from build123d import *

# Parameters (mm, degrees)
F2_R     = 11.5
F2_R_2   = 10
F3_DEPTH = 16
F4_DEPTH = 1.5
F5_R     = 0.3
F6_SIZE2 = 0.3
F6_SIZE  = 2


with BuildPart() as f3:
    # F2 (on Top) → F3 (new body)
    with BuildSketch(Plane.XY):
        Circle(F2_R)
        Circle(F2_R_2, mode=Mode.SUBTRACT)
    extrude(amount=F3_DEPTH)

    # F2 (on Top) → F4 (join)
    with BuildSketch(Plane.XY):
        Circle(F2_R_2)
    extrude(amount=F4_DEPTH)

    # F5
    f5_edges = [f3.edges().sort_by_distance(p)[0] for p in [
        (-11.5, 0, 0),
    ]]
    fillet(f5_edges, radius=F5_R)

    # F6
    f6_edges = [f3.edges().sort_by_distance(p)[0] for p in [
        (-10, 0, 16),
    ]]
    f6_side = f3.faces().sort_by_distance((-10, 0, 8.75))[0]
    chamfer(f6_edges, length=F6_SIZE, length2=F6_SIZE2, reference=f6_side)


solid = f3.part
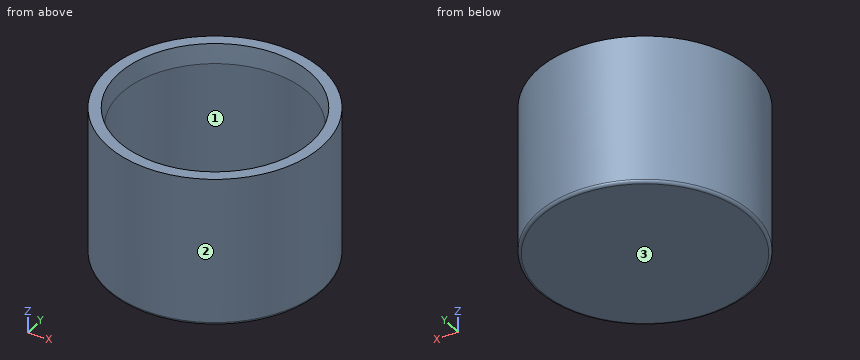
Could you check a few things on this model? Use its own coordinates, in mm. Face numbers are marked on the shaded views. Give positions to 0.01 mm unless a question says otherwise; leave off trailing zeros. Write each loop counter-clockwise with the first axis right and the second up, starting at its lowest first coordinate (ties: lowest second). Pieces come first, ordered by that corner, then holes. Notation, with made-up numbers: (-16.75, -5.5) -> (29.25, -5.5) arc R9 cw to (29.25, 6.5) -> close; hole circle Ø9 at (79.5, 62). An arc over 180 degrees is marked (long way). Answer as a JSON object with one key per item and string values.
Q1. Will these pins go through, and if not, where does the flat tip stop? pin 1 Ø2 at (x, z) = (-4.5, 12.5) entering from -Y; pin 2 Ø1.5 at (x, z) = (2, 1.5) entering from -Y; pin 3 Ø12 at (x, y) = (0, 0) entering from +Z.
Taken from the geometry:
{"pin 1": "stops at y = -10.95", "pin 2": "stops at y = -11.43", "pin 3": "stops at z = 1.5"}
Q2. Suppose I cut it at A-A on x = 0. Write out the boundary of the cut face in (y, z), then the cut area to 3 significant figures.
Taken from the geometry:
{"outline": "(-11.5, 0.3) arc R0.3 ccw to (-11.2, 0) -> (11.2, 0) arc R0.3 ccw to (11.5, 0.3) -> (11.5, 16) -> (10.3, 16) -> (10, 14) -> (10, 1.5) -> (-10, 1.5) -> (-10, 14) -> (-10.3, 16) -> (-11.5, 16) -> close", "area": "77.4 mm²"}
Q3. Suppose I cut it at C-C on z = 2.5. Write out the boundary of the cut face in (x, y), then the cut area to 3 significant figures.
Taken from the geometry:
{"outline": "circle Ø23 at (0, 0); hole circle Ø20 at (0, 0)", "area": "101 mm²"}
Q4. Please list where these lines run through material, in increasing order: L1, parallel to Y at x = 0, z = 7.25; L2, parallel to Z at x = 5.75, y = -4; L3, parallel to X at y = -5.75, z = 14.5.
Taken from the geometry:
{"L1": "y = -11.5 to -10, 10 to 11.5", "L2": "z = 0 to 1.5", "L3": "x = -9.96 to -8.27, 8.27 to 9.96"}
Q5. We'd pull the mould along Y, two halves only. Please class the marked faces 1, 2 and 3: released by +Y, released by -Y, zero draft, split by the parting line, or undercut.
Taken from the geometry:
{"face 1": "undercut", "face 2": "split by the parting line", "face 3": "zero draft"}
